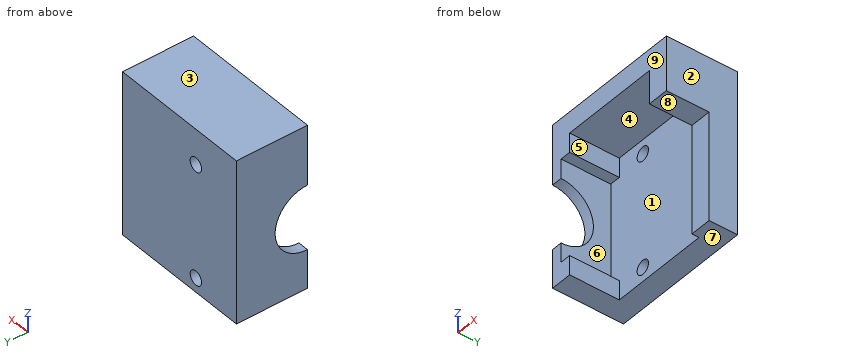
```python
from build123d import *

# Parameters (mm, degrees)
SKETCH1_W           = 20
SKETCH1_H           = 23
BOSS_EXTRUDE1_DEPTH = 10
CUT_EXTRUDE13_DEPTH = 7
SKETCH16_R          = 4.55
CUT_EXTRUDE14_DEPTH = 7
SKETCH18_W          = 14.55
SKETCH18_H          = 7
CUT_EXTRUDE16_DEPTH = 1.5
SKETCH20_R          = 1
CUT_EXTRUDE18_DEPTH = 5
SKETCH21_W          = 15.3
SKETCH21_H          = 6
CUT_EXTRUDE19_DEPTH = 5


with BuildPart() as part:
    # Sketch1 → Boss-Extrude1 (new body)
    with BuildSketch(Plane(origin=(0, 0, 0), x_dir=(1, 0, 0), z_dir=(0, 1, 0))):
        Rectangle(SKETCH1_W, SKETCH1_H)
    extrude(amount=BOSS_EXTRUDE1_DEPTH)

    # Sketch15 → Cut-Extrude13 (cut)
    with BuildSketch(Plane.XZ):
        Polygon((0, -11.5), (-7, -11.5), (-7, 8.5), (7, 8.5), (7, -11.5), align=None)
    extrude(amount=-CUT_EXTRUDE13_DEPTH, mode=Mode.SUBTRACT)

    # Sketch16 → Cut-Extrude14 (cut)
    with BuildSketch(Plane.ZY.offset(10)):
        with Locations((-1.5, 0)):
            Circle(SKETCH16_R)
    extrude(amount=-CUT_EXTRUDE14_DEPTH, mode=Mode.SUBTRACT)

    # Sketch18 → Cut-Extrude16 (cut)
    with BuildSketch(Plane(origin=(-7, 0, 0), x_dir=(0, 0, -1), z_dir=(1, 0, 0))):
        with Locations((1.5, 3.5)):
            Rectangle(SKETCH18_W, SKETCH18_H)
    extrude(amount=-CUT_EXTRUDE16_DEPTH, mode=Mode.SUBTRACT)

    # Sketch20 → Cut-Extrude18 (cut)
    with BuildSketch(Plane(origin=(0, 10, 0), x_dir=(1, 0, 0), z_dir=(0, 1, 0))):
        with Locations(Location((-2.88, 9.5, 0), (0, 0, 270))):
            Circle(SKETCH20_R)
        with Locations(Location((-2.88, -6.5, 0), (0, 0, 270))):
            Circle(SKETCH20_R)
    extrude(amount=-CUT_EXTRUDE18_DEPTH, mode=Mode.SUBTRACT)

    # Sketch21 → Cut-Extrude19 (cut)
    with BuildSketch(Plane(origin=(10, 0, 0), x_dir=(0, 0, -1), z_dir=(1, 0, 0))):
        with Locations((3.85, 3)):
            Rectangle(SKETCH21_W, SKETCH21_H)
    extrude(amount=-CUT_EXTRUDE19_DEPTH, mode=Mode.SUBTRACT)


solid = part.part
```
CAD build for the part. Positions are in the model's coordinates, mm. Face numbers are marked on the shaded views. A direction names the side the tool comes from. Round coordinates to 2 decimals unless told otherwise and drop trailing zeros. Write each loop counter-clockwise with the first axis right and the second up, starting at its lowest first coordinate (ties: lowest second). Pieces come first, ordered by that corner, then holes. Notation, with made-up numbers: (61.5, -15) - (95.5, -15) arc R19 ccw to (95.5, 13) - close; hole circle Ø9 at (82, -3.75). An arc over 180 degrees is marked (long way). Return JSON: item names as keys, results as strings. Group by question number.
Item 1: Band-saw the part on C-C on y = 3.5. List the corners of the cut face in (x, z) (3 decimals), plus the area to 3 significant figures.
Item 2: Mould opens along X. For the marked faces 1, 2, 3 and 4 say: +X half, -X half, draft (parallel to the pull), parting line (faces both ways), or undercut.
Item 3: Band-saw the part on A-A on z = -9.5. List the corners of the cut face in (x, y), plus the area to 3 significant figures.
Item 4: Band-saw the part on B-B on x = -2.88. List the corners of the cut face in (y, z).
Item 5: 3-axis set-ups, long thin cutter, end or side, ignore diameter. For the marked faces 5, 6, 7, 8 and 9: which of +Z, -Z, +X, -X, +Y, -Y reach the whole face in a straight line?
Item 6: Flat gauge pins, fed straight in: pin 1 Ø2 at (y, z) = (2, -10.5) entering from +X; pin 2 Ø0.9 at (x, y) = (8, 3.5) entering from -Z; pin 3 Ø2.5 at (x, z) = (-2.88, -9.5) entering from -Y. Where does each tip first touch, or does it go through?
Item 7: Band-saw the part on D-D on z = -1.5. List the corners of the cut face in (x, y), plus the area to 3 significant figures.
Item 8: Probe probe 1 along X at (y, z) = (8.6, -9.5); probe 2 along X at (y, z) = (6.5, 5); probe 3 along Z at (x, y) = (-3.5, 8). List the from-to ranges inside material, lowest first.
Resolved:
{
 "1": {"outline": "(-10, -11.5) - (-7, -11.5) - (-7, -8.775) - (-8.5, -8.775) - (-8.5, -4.407) - (-10, -4.407) - close; (-10, 1.407) - (-8.5, 1.407) - (-8.5, 5.775) - (-7, 5.775) - (-7, 8.5) - (7, 8.5) - (7, 3.8) - (10, 3.8) - (10, 11.5) - (-10, 11.5) - close", "area": "104 mm²"},
 "2": {"face 1": "undercut", "face 2": "+X half", "face 3": "draft", "face 4": "undercut"},
 "3": {"outline": "(-10, 0) - (-7, 0) - (-7, 7) - (-3.88, 7) - (-3.88, 10) - (-10, 10) - close; (-1.88, 7) - (7, 7) - (7, 6) - (10, 6) - (10, 10) - (-1.88, 10) - close", "area": "78.0 mm²"},
 "4": {"outline": "(0, 8.5) - (7, 8.5) - (7, 7.5) - (10, 7.5) - (10, 11.5) - (0, 11.5) - close; (7, -11.5) - (10, -11.5) - (10, -10.5) - (7, -10.5) - close; (7, -8.5) - (10, -8.5) - (10, 5.5) - (7, 5.5) - close"},
 "5": {"face 5": "-Z, -Y", "face 6": "-Y", "face 7": "-Z, +X, -X, +Y, -Y", "face 8": "-Z, +X, -Y", "face 9": "+Z, -Z, +X, -X, -Y"},
 "6": {"pin 1": "stops at x = -7", "pin 2": "stops at z = 3.8", "pin 3": "stops at y = 7"},
 "7": {"outline": "(-10, 4.55) - (-8.5, 4.55) - (-8.5, 7) - (7, 7) - (7, 6) - (10, 6) - (10, 10) - (-10, 10) - close", "area": "66.7 mm²"},
 "8": {"probe 1": "x = -10 to -3.88, -1.88 to 10", "probe 2": "x = -10 to -8.5, 7 to 10", "probe 3": "z = -11.5 to -10.28, -8.72 to 5.72, 7.28 to 11.5"}
}
